```python
from build123d import *

# Parameters (mm, degrees)
ESQUISSE1_W             = 30
ESQUISSE1_H             = 20
BOSS_EXTRU_1_DEPTH      = 2
ESQUISSE2_W             = 2
ESQUISSE2_H             = 20
BOSS_EXTRU_2_DEPTH      = 27
ENL_V_MAT_EXTRU_1_DEPTH = 27
ENL_V_MAT_EXTRU_2_DEPTH = 27
BOSS_EXTRU_3_DEPTH      = 2
BOSS_EXTRU_4_DEPTH      = 2
BOSS_EXTRU_5_DEPTH      = 3
CONG_2_R                = 0.5
CONG_3_R                = 0.5


with BuildPart() as part:
    # Esquisse1 → Boss.-Extru.1 (new body)
    with BuildSketch(Plane.XY):
        Rectangle(ESQUISSE1_W, ESQUISSE1_H)
    extrude(amount=BOSS_EXTRU_1_DEPTH)

    # Esquisse2 → Boss.-Extru.2 (add)
    with BuildSketch(Plane.XY.offset(2)):
        with Locations((-14, 0)):
            Rectangle(ESQUISSE2_W, ESQUISSE2_H)
    extrude(amount=BOSS_EXTRU_2_DEPTH)

    # Esquisse3 → Enlèv. mat.-Extru.1 (cut)
    with BuildSketch(Plane.XY.offset(2)):
        with BuildLine():
            Line((-2.5, 2), (2.5, 2))
            ThreePointArc((2.5, 2), (4.5, 0), (2.5, -2))
            Line((2.5, -2), (-2.5, -2))
            ThreePointArc((-2.5, -2), (-4.5, 0), (-2.5, 2))
        make_face()
    extrude(amount=-ENL_V_MAT_EXTRU_1_DEPTH, mode=Mode.SUBTRACT)

    # Esquisse4 → Enlèv. mat.-Extru.2 (cut)
    with BuildSketch(Plane(origin=(-13, 0, 0), x_dir=(0, 0, -1), z_dir=(1, 0, 0))):
        with BuildLine():
            Line((-18, 2), (-13, 2))
            ThreePointArc((-13, 2), (-11, 0), (-13, -2))
            Line((-13, -2), (-18, -2))
            ThreePointArc((-18, -2), (-20, 0), (-18, 2))
        make_face()
    extrude(amount=-ENL_V_MAT_EXTRU_2_DEPTH, mode=Mode.SUBTRACT)

    # Esquisse5 → Boss.-Extru.3 (add)
    with BuildSketch(Plane(origin=(0, -10, 0), x_dir=(-1, 0, 0), z_dir=(0, -1, 0))):
        Polygon((13, -29), (-15, -2), (13, -2), align=None)
    extrude(amount=-BOSS_EXTRU_3_DEPTH)

    # Esquisse6 → Boss.-Extru.4 (add)
    with BuildSketch(Plane(origin=(0, 10, 0), x_dir=(1, 0, 0), z_dir=(0, 1, 0))):
        Polygon((15, -2), (-13, -29), (-13, -2), align=None)
    extrude(amount=-BOSS_EXTRU_4_DEPTH)

    # Esquisse7 → Boss.-Extru.5 (add)
    with BuildSketch(Plane(origin=(0, 0, 0), x_dir=(-1, 0, 0), z_dir=(0, 0, -1))):
        with BuildLine():
            Line((-11.75, -1), (-11.75, 1))
            ThreePointArc((-11.75, 1), (-9.75, 3), (-7.75, 1))
            Line((-7.75, 1), (-7.75, -1))
            ThreePointArc((-7.75, -1), (-9.75, -3), (-11.75, -1))
        make_face()
        with BuildLine():
            Line((7.75, -1), (7.75, 1))
            ThreePointArc((7.75, 1), (9.75, 3), (11.75, 1))
            Line((11.75, 1), (11.75, -1))
            ThreePointArc((11.75, -1), (9.75, -3), (7.75, -1))
        make_face()
    extrude(amount=BOSS_EXTRU_5_DEPTH)

    # Congé2
    cong_2_edges = [part.edges().sort_by_distance(p)[0] for p in [
        (9.75, -3, -3),
        (7.75, 0, -3),
        (9.75, 3, -3),
        (11.75, 0, -3),
    ]]
    fillet(cong_2_edges, radius=CONG_2_R)

    # Congé3
    cong_3_edges = [part.edges().sort_by_distance(p)[0] for p in [
        (-9.75, -3, -3),
        (-11.75, 0, -3),
        (-9.75, 3, -3),
        (-7.75, 0, -3),
    ]]
    fillet(cong_3_edges, radius=CONG_3_R)


solid = part.part
```
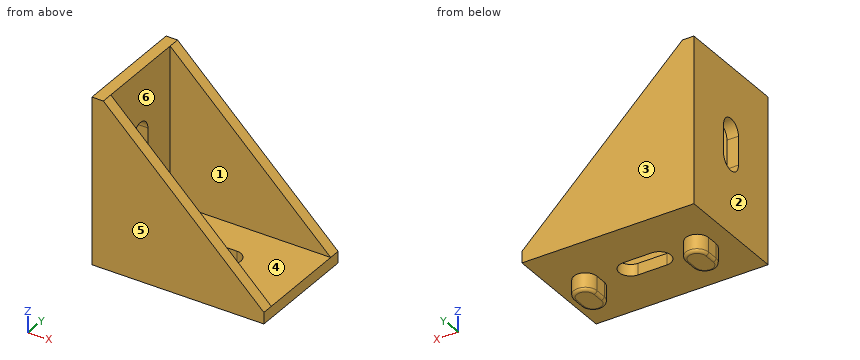
Source: CAD feature listing. Evaluate the final solid. Frame: model axes, mm. Face numbers are marked on the shaded views. A direction names the side the tool comes from. Round coordinates to 2 decimals unless told otherwise and drop trailing zeros. Order: outer loops, then holes, each group sorted by start corner. A loop starts at its lowest first (then second) coordinate and runs counter-clockwise, first axis right, second up. Notation, with made-up numbers: (70.25, 39.5) -> (107.25, 39.5) arc R21 ccw to (107.25, 64.5) -> close; hole circle Ø11 at (88, -32.5). An arc over 180 degrees is marked (long way). Use CSV: the item, a comma, the result in double quotes.
(1) Section A-A on y = 0. Return the cut outline in (x, z).
Report:
outline,"(-15, 0) -> (-11.75, 0) -> (-11.75, -2.5) arc R0.5 ccw to (-11.25, -3) -> (-8.25, -3) arc R0.5 ccw to (-7.75, -2.5) -> (-7.75, 0) -> (-4.5, 0) -> (-4.5, 2) -> (-13, 2) -> (-13, 11) -> (-15, 11) -> close; (-15, 20) -> (-13, 20) -> (-13, 29) -> (-15, 29) -> close; (4.5, 0) -> (7.75, 0) -> (7.75, -2.5) arc R0.5 ccw to (8.25, -3) -> (11.25, -3) arc R0.5 ccw to (11.75, -2.5) -> (11.75, 0) -> (15, 0) -> (15, 2) -> (4.5, 2) -> close"
(2) Access query for the marked faces 1 and 2. Directions: +Z, -Z, +X, -X, +Y, -Y. A direction counts if a zero-diameter tool reaches every point of the face in a straight line with its end or side. Return the directions, or none.
Report:
face 1,"+Z, +X"
face 2,"+Z, -Z, -X, +Y, -Y"
(3) First-contact query: pin 1 Ø1.6 at (y, z) = (0.5, -1) entering from -X; pin 2 Ø6 at (x, y) = (5.5, -4) entering from +Z; pin 3 Ø2 at (y, z) = (2, 19) entering from +X. Flat tips, straight axial feed; report the tip coordinate or a pass-through.
Report:
pin 1,"x = -11.75"
pin 2,"z = 2"
pin 3,"x = -13"
(4) Section D-D on y = 4.75. Return the cut outline in (x, z).
Report:
outline,"(-15, 0) -> (15, 0) -> (15, 2) -> (-13, 2) -> (-13, 29) -> (-15, 29) -> close"
(5) Section B-B on x = 0.25. Return the cut outline in (y, z), and give its area (3 significant figures).
Report:
outline,"(-10, 0) -> (-2, 0) -> (-2, 2) -> (-8, 2) -> (-8, 16.22) -> (-10, 16.22) -> close; (2, 0) -> (10, 0) -> (10, 16.22) -> (8, 16.22) -> (8, 2) -> (2, 2) -> close"
area,"88.9 mm^2"
(6) Pull-direction query (Y, two-part tool) for the marked faces 3, 4, 5 and 6; classes: +Y half, -Y half, draft (parallel to the pull), parting line (faces both ways), or undercut.
Report:
face 3,"+Y half"
face 4,"undercut"
face 5,"-Y half"
face 6,"undercut"
(7) Section C-C on z = 24.5. Return the cut outline in (x, y), and give its area (3 significant figures).
Report:
outline,"(-15, -10) -> (-8.33, -10) -> (-8.33, -8) -> (-13, -8) -> (-13, 8) -> (-8.33, 8) -> (-8.33, 10) -> (-15, 10) -> close"
area,"58.7 mm^2"
(8) Ray query, L1, parallel to Y at x = -8.25, z = 21.5; L2, parallel to Z at x = 8.5, y = 6.5; L3, parallel to X at y = 5, z = 20.5. Return the intervals inside material, ascending.
Report:
L1,"-10 to -8, 8 to 10"
L2,"0 to 2"
L3,"-15 to -13"
